Autodesk Inventor part; units mm, degrees
ref_plane "YZ Plane" through (0, 0, 0) normal (1, 0, 0) x (0, 1, 0)
ref_plane "XZ Plane" through (0, 0, 0) normal (0, 1, 0) x (-1, 0, 0)
ref_plane "XY Plane" through (0, 0, 0) normal (0, 0, 1) x (1, 0, 0)
sketch "Sketch1" plane through (0, 0, 0) normal (0, 1, 0) x (-1, 0, 0)
  line L0 (15.5801, 16.9856) -> (11.25, 19.4856)
  line L1 (11.25, -19.4856) -> (15.5801, -16.9856)
  line L2 (11.25, 19.4856) -> (0, 0)
  line L3 (0, 0) -> (11.25, -19.4856)
  line L4 (15.5801, 16.9856) -> (15.5801, -16.9856)
  circle A0 centre (5.625, 0) radius 1.4
  circle A1 centre (11.25, -9.7428) radius 1.4
  circle A2 centre (11.25, 9.7428) radius 1.4
  dimension "d4" = 2.8
  dimension "d5" = 2.8
  dimension "d6" = 2.8
extrude "Extrusion1" add sketch "Sketch1" along normal blind 50
sketch "Sketch3" plane through (0, 50, 0) normal (0, 1, 0) x (1, 0, 0)
  circle A0 centre (-11.25, -9.7428) radius 1.4
  circle A1 centre (-11.25, 9.7428) radius 1.4
  circle A2 centre (-5.625, 0) radius 1.4
  line L0 (-15.5801, -16.9856) -> (-11.25, -19.4856)
  line L1 (-11.25, -19.4856) -> (0, 0)
  line L2 (0, 0) -> (-11.25, 19.4856)
  line L3 (-11.25, 19.4856) -> (-15.5801, 16.9856)
  line L4 (-15.5801, 16.9856) -> (-15.5801, -16.9856)
  line L5 (-11.25, 0) -> (-15.5801, 16.9856)
  line L6 (-11.25, 0) -> (-15.5801, -16.9856)
  dimension "d15" = 5.625
extrude "Extrusion3" add sketch "Sketch3" against normal blind 40 contours A0 | A1 | A2 | L4 L5 L6
sketch "Sketch4" plane through (0, 50, 0) normal (0, 1, 0) x (1, 0, 0)
  line L0 (-11.25, -19.4856) -> (-5.25, -19.4856) construction
  circle A0 centre (-12.2919, -13.5767) radius 1.4
  line L1 (0, 0) -> (-15.5801, 0)
  line L2 (-15.5801, 16.9856) -> (-15.5801, -16.9856)
  circle A1 centre (-12.2919, 13.5767) radius 1.4
  circle A2 centre (-12.2919, 13.5767) radius 2.75
  circle A3 centre (-12.2919, -13.5767) radius 2.75
  point P0 (-11.25, 19.4856)
  dimension "d12" = 2.8
  dimension "d78" = 5.5
  dimension "d79" = 5.5
extrude "Extrusion4" add sketch "Sketch4" along normal blind 30
sketch "Sketch6" plane through (-15.5801, 0, -16.9856) normal (-1, 0, 0) x (0, 0, 1)
  line L0 (16.9856, 15) -> (16.9856, 20)
  line L1 (16.9856, 50) -> (16.9856, 23)
  line L2 (16.9856, 20) -> (6.9856, 20)
  line L3 (26.9856, 20) -> (16.9856, 20)
  line L4 (6.9856, 20) -> (8.4856, 20)
  line L5 (8.4856, 20) -> (8.4856, 21.5)
  line L6 (26.9856, 20) -> (25.4856, 20)
  line L7 (25.4856, 20) -> (25.4856, 21.5)
  circle A0 centre (25.4856, 21.5) radius 0.6
  circle A1 centre (8.4856, 21.5) radius 0.6
  line L8 (16.9856, 20) -> (16.9856, 29)
  circle A2 centre (16.9856, 29) radius 8.5
  line L9 (16.9856, 29) -> (16.9856, 56)
  circle A3 centre (16.9856, 56) radius 8.5
  line L10 (26.9856, 20) -> (26.9856, 65)
  line L11 (26.9856, 65) -> (6.9856, 65)
  line L12 (6.9856, 65) -> (6.9856, 20)
  point P0 (16.9856, 0)
  dimension "d23" = 5
  dimension "d24" = 10
  dimension "d28" = 1.5
  dimension "d29" = 1.5
  dimension "d30" = 1.5
  dimension "d31" = 1.5
  dimension "d32" = 1.2
  dimension "d33" = 1.2
  dimension "d34" = 9
  dimension "d35" = 17
  dimension "d36" = 27
  dimension "d37" = 17
  dimension "d38" = 45
  dimension "d39" = 20
extrude "Extrusion6" cut sketch "Sketch6" against normal through all contours L1 A2 L8 | L1 L8 A2 | A3
sketch "Sketch7" plane through (-15.5801, 0, -16.9856) normal (-1, 0, 0) x (0, 0, 1)
  line L0 (16.9856, 15) -> (16.9856, 20)
  line L1 (16.9856, 50) -> (16.9856, 15)
  line L2 (16.9856, 20) -> (6.9856, 20)
  line L3 (26.9856, 20) -> (16.9856, 20)
  line L4 (6.9856, 20) -> (8.4856, 20)
  line L5 (8.4856, 20) -> (8.4856, 21.5)
  line L6 (26.9856, 20) -> (25.4856, 20)
  line L7 (25.4856, 20) -> (25.4856, 21.5)
  circle A0 centre (25.4856, 21.5) radius 0.9
  circle A1 centre (8.4856, 21.5) radius 0.9
  line L8 (16.9856, 20) -> (16.9856, 29)
  circle A2 centre (16.9856, 29) radius 8.5
  line L9 (16.9856, 29) -> (16.9856, 56)
  circle A3 centre (16.9856, 56) radius 8.5
  line L10 (26.9856, 20) -> (26.9856, 65)
  line L11 (26.9856, 65) -> (6.9856, 65)
  line L12 (6.9856, 65) -> (6.9856, 20)
  point P0 (16.9856, 0)
  point P1 (16.9856, 0)
  dimension "d42" = 5
  dimension "d43" = 10
  dimension "d44" = 1.5
  dimension "d45" = 1.5
  dimension "d46" = 1.5
  dimension "d47" = 1.5
  dimension "d48" = 1.8
  dimension "d49" = 1.8
  dimension "d50" = 9
  dimension "d51" = 17
  dimension "d52" = 27
  dimension "d53" = 17
  dimension "d54" = 45
  dimension "d55" = 20
extrude "Extrusion7" cut sketch "Sketch7" against normal blind 9 contours A0 | A1
sketch "Sketch8" plane through (-15.5801, 0, -16.9856) normal (-1, 0, 0) x (0, 0, 1)
  line L0 (5.9856, 20) -> (5.9856, 19)
  line L1 (28.0623, 50) -> (28.0623, 80)
  line L2 (26.9856, 66) -> (27.9856, 66)
  line L3 (27.9856, 66) -> (5.9856, 66)
  line L4 (5.9856, 66) -> (5.9856, 19)
  line L5 (5.9856, 19) -> (27.9856, 19)
  line L6 (27.9856, 19) -> (27.9856, 66)
  point P0 (16.9856, 0)
  point P1 (16.9856, 15)
  dimension "d73" = 1
  dimension "d75" = 1
extrude "Extrusion8" cut sketch "Sketch8" against normal blind 2
properties part number "Support" material "ABS Plastic"
Design review of the part built by this model. Coordinates are the model's own, in mm. A direction names the side the tool comes from. Coordinates: 2 decimals unless noted, no trailing zeros. Order: outer loops, then holes, each group sorted by start corner. A loop starts at its lowest first (then second) coordinate and runs counter-clockwise, first axis right, second up. Notation, with made-up numbers: M 0.25,-8.75 L 11.25,-8.75 A21 cw 11.25,30.25 Z; hole C -4,24 d11. An arc over 180 degrees is marked long. Use a Markdown table: item, result.
(1) Draft analysis for pull direction Z (two halves, no side actions). For faces 1 (the flat face through (-14, 80, 13)), 2 (the flat face through (-5.55, 24.65, -9.61)), 3 (the flat face through (-11, 10, 10)), state which applies: released by +Z, released by -Z, zero draft, split by the parting line, or undercut.
Worked answers:
| item | result |
|---|---|
| face 1 | zero draft |
| face 2 | released by -Z |
| face 3 | undercut |
(2) Add section B-B (z = -5). Give the boundary of the cut face in (x, y).
Worked answers:
| item | result |
|---|---|
| outline | M -15.58,0 L -2.89,0 L -2.89,22.13 L -13.58,22.13 L -13.58,19 L -15.58,19 Z; M -13.58,35.87 L -2.89,35.87 L -2.89,49.13 L -13.58,49.13 Z |
(3) Add section C-C (y = 29). Give the boundary of the cut face in (x, z), then the cut area to 3 significant figures.
Worked answers:
| item | result |
|---|---|
| outline | M -15.58,-16.99 L -11.25,-19.49 L -4.91,-8.5 L -13.58,-8.5 L -13.58,-11 L -15.58,-11 Z; M -15.58,11 L -13.58,11 L -13.58,8.5 L -4.91,8.5 L -11.25,19.49 L -15.58,16.99 Z |
| area | 144 mm2 |
(4) Add section D-D (y = 58). Give the boundary of the cut face in (x, z).
Worked answers:
| item | result |
|---|---|
| outline | C -12.29,-13.58 d5.5; C -12.29,13.58 d5.5; hole C -12.29,-13.58 d2.8; hole C -12.29,13.58 d2.8 |
(5) Wall thickness on probe 1 along Y at (x, z) = (-7.5, 0); probe 2 along Y at (x, z) = (-6.5, -7.5); probe 3 along Z at (x, y) = (-6.5, 29): over which ranges is each line inside the solid? List them lowest first.
Worked answers:
| item | result |
|---|---|
| probe 1 | y = 0 to 20.5, 37.5 to 47.5 |
| probe 2 | y = 0 to 25, 33 to 50 |
| probe 3 | z = -11.26 to -8.5, 8.5 to 11.26 |
(6) Add section A-A (y = 17). Give the boundary of the cut face in (x, z), then the cut area to 3 significant figures.
Worked answers:
| item | result |
|---|---|
| outline | M -15.58,-16.99 L -11.25,-19.49 L 0,0 L -11.25,19.49 L -15.58,16.99 Z |
| area | 377 mm2 |
(7) For P1, Ø3, axis at y = 22.5, z = -6.5, coming from the +X side; P2, Ø11, axis at y = 38, z = 5, coming from the -X side; P3, Ø5, axis at x = -9.5, y = 39.5, coming from the +Z side, all flat-tipped, find the tip position at first contact; note any pin that passes through.
Worked answers:
| item | result |
|---|---|
| P1 | stops at x = -2.91 |
| P2 | stops at x = -13.58 |
| P3 | stops at z = 19.49 |
(8) For faces 4 (the flat face through (-12, 50, -14)), 5 (the flat face through (-15.58, 14, 0)), 6 (the cylindrical face through (-6.96, 4.93, -0.42)), 7 (the flat face through (-15, 19, 0)), 8 (the flat face through (-13.445, 24.65, 18.218)), list the 3-axis set-ups (+Z, -Z, +X, -X, +Y, -Y) from which the entire face can be reached by the end or side of a thin tool; tool diameter is ignored.
Worked answers:
| item | result |
|---|---|
| face 4 | +Y |
| face 5 | +Z, -Z, -X, +Y, -Y |
| face 6 | -Y |
| face 7 | -X, +Y |
| face 8 | +Z, -X, +Y, -Y |
